```python
from build123d import *

# Parameters (mm, degrees)
SKETCH1_R           = 1.5
BOSS_EXTRUDE1_DEPTH = 197
SKETCH2_W           = 0.5
SKETCH2_H           = 0.25


with BuildPart() as part:
    # Sketch1 → Boss-Extrude1 (new body)
    with BuildSketch(Plane(origin=(0, 0, 0), x_dir=(0, 0, -1), z_dir=(1, 0, 0))):
        Circle(SKETCH1_R)
    extrude(amount=BOSS_EXTRUDE1_DEPTH)

    # Sketch2 → Cut-Revolve1 (revolve, cut)
    with BuildSketch(Plane.XY, mode=Mode.PRIVATE) as cut_revolve1_sk:
        with Locations((1.55, 1.375)):
            Rectangle(SKETCH2_W, SKETCH2_H)
    cut_revolve1 = revolve(cut_revolve1_sk.sketch.rotate(Axis((197, 0, 0), (-1, 0, 0)), 90), axis=Axis((197, 0, 0), (-1, 0, 0)), mode=Mode.SUBTRACT)

    # Mirror1: Cut-Revolve1 across plane
    add(cut_revolve1.mirror(Plane.ZY.offset(-98.5)), mode=Mode.SUBTRACT)


solid = part.part
```
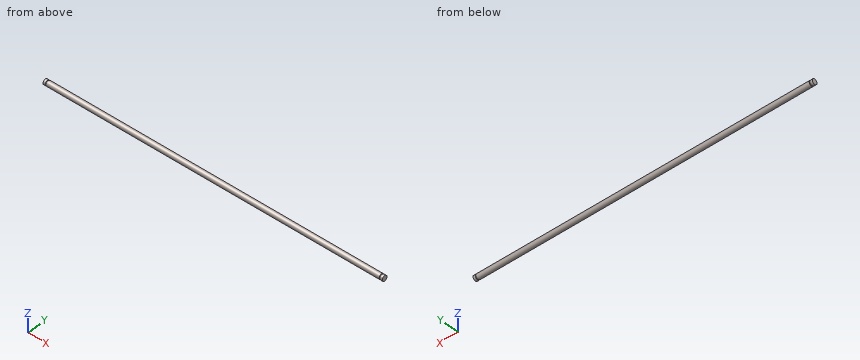
Part model, mm, in its own coordinate system. Round coordinates to 2 decimals unless told otherwise and drop trailing zeros. Order: outer loops, then holes, each group sorted by start corner. A loop starts at its lowest first (then second) coordinate and runs counter-clockwise, first axis right, second up. Notation, with made-up numbers: M 20.25,-11 L 55.25,-11 A18 cw 55.25,8 Z; hole C 27.25,40.25 d1. An arc over 180 degrees is marked long. Answer in a Markdown table with one row per item. Add a question column.
Q1. Cut at A-A on x = 140. Give the cut face in (y, z).
Q2. Wall check: L1, parallel to X at y = -0.6, z = -1.3; L2, parallel to Y at x = 8, z = -0.2; L3, parallel to Z at x = 163, y = -0.8. Give the ranges that are in metal, low to high. Write a range as from..to.
Q3. Cut at B-B on z = -0.8. Give the cut face in (x, y), and give its area (3 significant figures).
Established:
| question | item | result |
|---|---|---|
| 1 | outline | C 0,0 d3 |
| 2 | L1 | x = 0..1.3, 1.8..195.2, 195.7..197 |
| 2 | L2 | y = -1.49..1.49 |
| 2 | L3 | z = -1.27..1.27 |
| 3 | outline | M 0,-1.27 L 1.3,-1.27 L 1.3,-0.96 L 1.8,-0.96 L 1.8,-1.27 L 195.2,-1.27 L 195.2,-0.96 L 195.7,-0.96 L 195.7,-1.27 L 197,-1.27 L 197,1.27 L 195.7,1.27 L 195.7,0.96 L 195.2,0.96 L 195.2,1.27 L 1.8,1.27 L 1.8,0.96 L 1.3,0.96 L 1.3,1.27 L 0,1.27 Z |
| 3 | area | 499 mm2 |
